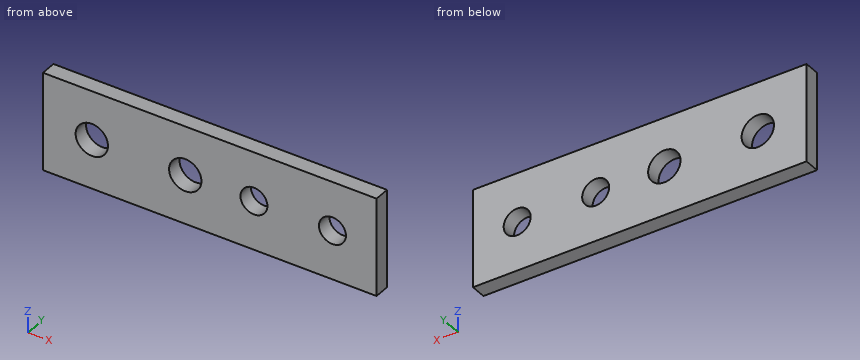
from build123d import *

# Parameters (mm, degrees)
SKETCH1_W                = 68
SKETCH1_H                = 20
BOSS_EXTRUDE1_DEPTH      = 3.175
M6_CLEARANCE_HOLE1_D     = 6.6
M6_CLEARANCE_HOLE1_DEPTH = 14
M6_CLEARANCE_HOLE1_TIP   = 1.982840043
M5_CLEARANCE_HOLE1_D     = 5.5
M5_CLEARANCE_HOLE1_DEPTH = 14
M5_CLEARANCE_HOLE1_TIP   = 1.652366702


with BuildPart() as part:
    # Sketch1 → Boss-Extrude1 (new body)
    with BuildSketch(Plane(origin=(0, 0, 0), x_dir=(1, 0, 0), z_dir=(0, 1, 0))):
        with Locations((-34, 10)):
            Rectangle(SKETCH1_W, SKETCH1_H)
    extrude(amount=BOSS_EXTRUDE1_DEPTH)

    # M6 Clearance Hole1
    with Locations(Plane(origin=(-39, 3.175, -10), x_dir=(0, 0, 1), z_dir=(0, 1, 0))):
        with Locations((0, 0), (0, -19.05)):
            Hole(M6_CLEARANCE_HOLE1_D / 2, depth=M6_CLEARANCE_HOLE1_DEPTH)
            with Locations((0, 0, -(M6_CLEARANCE_HOLE1_DEPTH + M6_CLEARANCE_HOLE1_TIP / 2))):  # 118° drill point
                Cone(0, M6_CLEARANCE_HOLE1_D / 2, M6_CLEARANCE_HOLE1_TIP, mode=Mode.SUBTRACT)

    # M5 Clearance Hole1
    with Locations(Plane(origin=(-25, 3.175, -10), x_dir=(0, 0, 1), z_dir=(0, 1, 0))):
        with Locations((0, 0), (0, 16)):
            Hole(M5_CLEARANCE_HOLE1_D / 2, depth=M5_CLEARANCE_HOLE1_DEPTH)
            with Locations((0, 0, -(M5_CLEARANCE_HOLE1_DEPTH + M5_CLEARANCE_HOLE1_TIP / 2))):  # 118° drill point
                Cone(0, M5_CLEARANCE_HOLE1_D / 2, M5_CLEARANCE_HOLE1_TIP, mode=Mode.SUBTRACT)


solid = part.part
Check sheet for the modelled part. Datum: model origin and axes. Units: mm. Round coordinates to 2 decimals unless told otherwise and drop trailing zeros. Loops run counter-clockwise (first coordinate to the right, second up) from the corner with the lowest first, then second, coordinate; pieces in that order, holes last. Notation, with made-up numbers: M 62.25,-17 L 101.25,-17 A28 ccw 101.25,8 Z; hole C 65.25,59 d5. An arc over 180 degrees is marked long. One line per item, written item: value.
(1) Sectioned sample at C-C, the plane z = -10. Record the cut outline in (x, y) (3 decimals).
Computed values:
outline: M -68,0 L -61.35,0 L -61.35,3.175 L -68,3.175 Z; M -54.75,0 L -42.3,0 L -42.3,3.175 L -54.75,3.175 Z; M -35.7,0 L -27.75,0 L -27.75,3.175 L -35.7,3.175 Z; M -22.25,0 L -11.75,0 L -11.75,3.175 L -22.25,3.175 Z; M -6.25,0 L 0,0 L 0,3.175 L -6.25,3.175 Z
(2) Sectioned sample at D-D, the plane x = -9. Record the cut outline in (y, z) (3 decimals).
Computed values:
outline: M 0,-20 L 3.175,-20 L 3.175,-12.75 L 0,-12.75 Z; M 0,-7.25 L 3.175,-7.25 L 3.175,0 L 0,0 Z
(3) Sectioned sample at A-A, the plane x = -58.05. Record the cut outline in (y, z) (3 decimals).
Computed values:
outline: M 0,-20 L 3.175,-20 L 3.175,-13.3 L 0,-13.3 Z; M 0,-6.7 L 3.175,-6.7 L 3.175,0 L 0,0 Z
(4) Thickness scan on line 1 (X direction, y = 1.85, z = -10); line 2 (X direction, y = 2.6, z = -11); line 3 (Z direction, x = -36, y = 2.8). Record the ranges inside material, lowest first.
Computed values:
line 1: x = -68 to -61.35, -54.75 to -42.3, -35.7 to -27.75, -22.25 to -11.75, -6.25 to 0
line 2: x = -68 to -61.19, -54.91 to -42.14, -35.86 to -27.56, -22.44 to -11.56, -6.44 to 0
line 3: z = -20 to -11.37, -8.63 to 0
(5) Sectioned sample at B-B, the plane y = 2.6. Record the cut outline in (x, z).
Computed values:
outline: M -68,-20 L 0,-20 L 0,0 L -68,0 Z; hole C -58.05,-10 d6.6; hole C -39,-10 d6.6; hole C -25,-10 d5.5; hole C -9,-10 d5.5
